Solid Edge part; units mm, degrees
sketch "Sketch1" plane through (0, 0, 0) normal (0, -1, 0) x (1, 0, 0)
  line L0 (3.5, 4) -> (3.5, 0)
  line L1 (3.5, 0) -> (2.35, 0)
  line L2 (2.35, 0) -> (2, -0.6062)
  line L3 (2, -0.6062) -> (2, -15)
  line L4 (2, -15) -> (0, -15)
  line L5 (1.5, 2) -> (0, 1.834)
  line L6 (1.5, 4) -> (1.5, 2)
  line L7 (3.5, 4) -> (1.5, 4)
revolve "RevolvedProtrusion1" add sketch "Sketch1" angle 360 about axis through (0, 0, -6) along (0, 0, 1)
cosmetic_thread "Thread1"
chamfer "Chamfer_1" distance 0.4 angle 45 1 edges at (-2, 0, -15)
fillet "Round_1" radius 0.4 2 edges at (-3.5, 0, 0) (-3.5, 0, 4)
sketch "Sketch2" plane through (0, 0, 4) normal (0, 0, 1) x (0, 1, 0)
  line L0 (-1.5, 0.866) -> (-1.5, -0.866)
  line L1 (0, -1.7321) -> (-1.5, -0.866)
  line L2 (1.5, -0.866) -> (0, -1.7321)
  line L3 (1.5, 0.866) -> (1.5, -0.866)
  line L4 (0, 1.7321) -> (1.5, 0.866)
  line L5 (-1.5, 0.866) -> (0, 1.7321)
extrude "Cutout1" cut sketch "Sketch2" against normal up to vertex (2 mm away)
properties material "Galvanized steel"
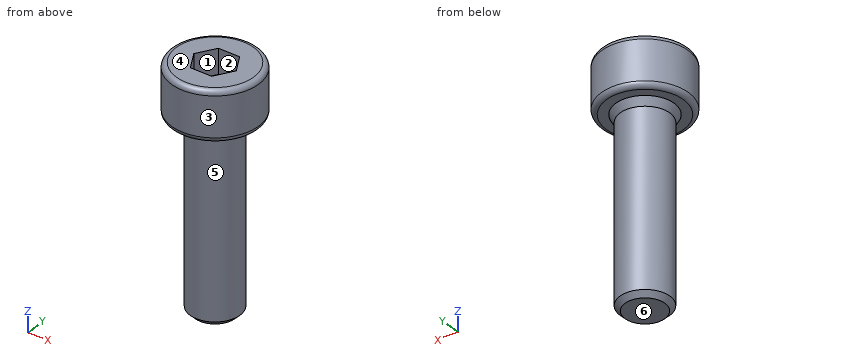
Geometry: final body of the model. Coordinates: model frame, mm. Face numbers are marked on the shaded views. A direction names the side the tool comes from. Give positions to 0.01 mm unless a question says otherwise; leave off trailing zeros. Loops run counter-clockwise (first coordinate to the right, second up) from the corner with the lowest first, then second, coordinate; pieces in that order, holes last. Notation, with made-up numbers: (22.25, 37.5) - (81.25, 37.5) arc R15 ccw to (81.25, 48.5) - close; hole circle Ø2 at (61.5, 15). An arc over 180 degrees is marked (long way). Answer as CSV lines item,"result". Start each with the question number.
1. Section B-B, the plane z = -8. Return loops of the section in (x, y), plus the area to 3 significant figures.
2. Ray query, L1, parallel to Z at x = 2.75, y = 1.5; L2, parallel to X at y = -1, z = -10; L3, parallel to X at y = -1.5, z = -5.75. Return the intervals inside material, ascending.
3. Section A-A, the plane z = 2.75. Return loops of the section in (x, y).
4. Pin query (flat end, axial travel): P1, Ø1, axis at y = -1, z = -4.5, coming from the +X side; P2, Ø1.5, axis at x = 2.5, y = -2, coming from the -Z side; P3, Ø0.5, axis at x = 0.5, y = -0.5, coming from the +Z side. Return the tip coordinate at first contact, or that it passes through.
5. Reachability of the marked faces 5 and 6 from +Z, -Z, +X, -X, +Y, -Y: full face, straight path, thin tool, end or side. Return the list, or none.
6. Draft query along X for the marked faces 1, 2, 3 and 4. Return one class per face: released by +X, released by -X, zero draft, split by the parting line, or undercut.
Answers:
1,outline,"circle Ø4 at (0, 0)"
1,area,"12.6 mm2"
2,L1,"z = 0 to 4"
2,L2,"x = -1.73 to 1.73"
2,L3,"x = -1.32 to 1.32"
3,outline,"circle Ø7 at (0, 0); hole (-1.73, 0) - (-0.87, -1.5) - (0.87, -1.5) - (1.73, 0) - (0.87, 1.5) - (-0.87, 1.5) - close"
4,P1,"stops at x = 1.94"
4,P2,"stops at z = 0"
4,P3,"stops at z = 1.94"
5,face 5,"-Z"
5,face 6,"-Z, +X, -X, +Y, -Y"
6,face 1,"undercut"
6,face 2,"undercut"
6,face 3,"split by the parting line"
6,face 4,"zero draft"
